The model under review builds one solid part; all positions refer to its coordinate system, in mm. A direction names the side the tool comes from. Coordinates: 2 decimals unless noted, no trailing zeros. Write each loop counter-clockwise with the first axis right and the second up, starting at its lowest first coordinate (ties: lowest second). Pieces come first, ordered by that corner, then holes. Notation, with made-up numbers: (58.5, 16.25) - (82.5, 16.25) arc R23 cw to (82.5, 42.25) - close; hole circle Ø1 at (66.25, 78). An arc over 180 degrees is marked (long way). Put each result on its own line as item: value.
Autodesk Inventor part; units mm, degrees
ref_plane "YZ Plane" through (0, 0, 0) normal (1, 0, 0) x (0, 1, 0)
ref_plane "XZ Plane" through (0, 0, 0) normal (0, 1, 0) x (-1, 0, 0)
ref_plane "XY Plane" through (0, 0, 0) normal (0, 0, 1) x (1, 0, 0)
sketch "Sketch1" plane through (0, 0, 0) normal (0, 1, 0) x (-1, 0, 0)
  line L0 (217.5, -122.5) -> (-217.5, -122.5)
  line L1 (-217.5, -122.5) -> (-217.5, 122.5)
  line L2 (-217.5, 122.5) -> (217.5, 122.5)
  line L3 (217.5, 122.5) -> (217.5, -122.5)
  line L4 (217.5, -122.5) -> (-217.5, 122.5) construction
  line L5 (-217.5, -122.5) -> (217.5, 122.5) construction
  point P0 (0, 0)
  dimension "d0" = 435
  dimension "d1" = 245
extrude "Extrusion1" add sketch "Sketch1" along normal blind 145
sketch "Sketch3" plane through (217.5, 0, 122.5) normal (1, 0, 0) x (0, 0, -1)
  line L0 (73, 65) -> (172, 65)
  line L1 (172, 65) -> (172, 20)
  line L2 (172, 20) -> (73, 20)
  line L3 (73, 20) -> (73, 65)
  line L4 (245, 0) -> (245, 145)
  line L5 (0, 145) -> (245, 145)
  line L6 (0, 5) -> (240, 5)
  point P0 (122.5, 0)
  point P1 (172, 42.5)
  dimension "d12" = 73
  dimension "d13" = 80
  dimension "d14" = 99
  dimension "d16" = 45
extrude "Extrusion3" cut sketch "Sketch3" against normal blind 450
sketch "Sketch4" plane through (0, 145, 0) normal (0, 1, 0) x (1, 0, 0)
  line L0 (-208, 113) -> (208, 113)
  line L1 (208, 113) -> (208, -113)
  line L2 (208, -113) -> (-208, -113)
  line L3 (-208, -113) -> (-208, 113)
  line L4 (217.5, 122.5) -> (-217.5, 122.5)
  line L5 (217.5, -122.5) -> (217.5, 122.5)
  line L6 (-217.5, -122.5) -> (217.5, -122.5)
  line L7 (-217.5, 122.5) -> (-217.5, -122.5)
  point P0 (0, 0)
  dimension "d19" = 9.5
  dimension "d20" = 9.5
  dimension "d21" = 9.5
  dimension "d22" = 9.5
extrude "Extrusion4" cut sketch "Sketch4" against normal blind 137 contours L0 L1 L2 L3
properties part number "Kenyertarto"
1. Machinability: for faces 4 (the flat face through (208, 77, -2)), 5 (the flat face through (-213, 43, -49.5)), 6 (the flat face through (17, 145, -117)), which of the approach directions +Z, -Z, +X, -X, +Y, -Y give a long, thin tool a straight path to every point of the face, cutting with its end or side? Answer none if there is none.
Determined:
face 4: +Y
face 5: +X, -X
face 6: +Z, -Z, +X, -X, +Y
2. Consider section B-B on z = 11. State the section outline as (x, y) points, plus the area to 3 significant figures.
Determined:
outline: (-217.5, 0) - (217.5, 0) - (217.5, 20) - (208, 20) - (208, 8) - (-208, 8) - (-208, 20) - (-217.5, 20) - close; (-217.5, 65) - (-208, 65) - (-208, 145) - (-217.5, 145) - close; (208, 65) - (217.5, 65) - (217.5, 145) - (208, 145) - close
area: 5,230 mm^2
3. The part is to be moulded in two halves that separate along Z. For faces 1 (the flat face through (-3, 77, -113)), 2 (the flat face through (3, 0, 2)), 3 (the flat face through (3, 71, 122.5)), say which applies: +Z half, -Z half, draft (parallel to the pull), parting line (faces both ways), or undercut.
Determined:
face 1: undercut
face 2: draft
face 3: +Z half
4. Consider section C-C on x = -80. State the section outline as (y, z) points.
Determined:
outline: (0, -122.5) - (145, -122.5) - (145, -113) - (8, -113) - (8, 113) - (145, 113) - (145, 122.5) - (0, 122.5) - close
5. Consider section A-A on y = 58.5. State the section outline as (x, z) points.
Determined:
outline: (-217.5, -122.5) - (217.5, -122.5) - (217.5, -49.5) - (208, -49.5) - (208, -113) - (-208, -113) - (-208, -49.5) - (-217.5, -49.5) - close; (-217.5, 49.5) - (-208, 49.5) - (-208, 113) - (208, 113) - (208, 49.5) - (217.5, 49.5) - (217.5, 122.5) - (-217.5, 122.5) - close
6. For pin 1 Ø7.5 at (x, z) = (213.5, -22.5) entering from -Y; pin 2 Ø4 at (x, z) = (-158.5, 4) entering from +Y, all flat-tipped, find the tip position at first contact; note any pin that passes through.
Determined:
pin 1: stops at y = 0
pin 2: stops at y = 8
7. To check wall thickness, follow probe 1 along Z at (x, y) = (10.5, 138.5); probe 2 along X at (y, z) = (120.5, -70.5); probe 3 along Y at (x, z) = (-0.5, 106). State the ranges of each line that lie inside material, in increasing order.
Determined:
probe 1: z = -122.5 to -113, 113 to 122.5
probe 2: x = -217.5 to -208, 208 to 217.5
probe 3: y = 0 to 8
8. Consider section D-D on z = 103. State the section outline as (x, y) points, plus the area to 3 significant figures.
Determined:
outline: (-217.5, 0) - (217.5, 0) - (217.5, 145) - (208, 145) - (208, 8) - (-208, 8) - (-208, 145) - (-217.5, 145) - close
area: 6,080 mm^2
